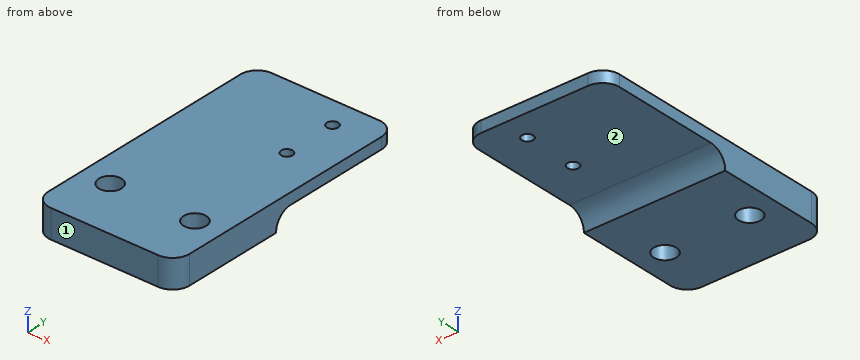
from build123d import *

# Parameters (mm, degrees)
SKETCH_1_W          = 25
SKETCH_1_H          = 46
EXTRUDE_1_DEPTH     = 5
SKETCH_2_W          = 25
SKETCH_2_H          = 25
CUT_EXTRUDE_1_DEPTH = 3
M4X0_7_1_D          = 4
M2X0_4_1_D          = 2
FILLET_1_R          = 3
FILLET_2_R          = 3


with BuildPart() as part:
    # ｽｹｯﾁ1 → ﾎﾞｽ - 押し出し1 (new body)
    with BuildSketch(Plane.XY):
        with Locations((12.5, 23)):
            Rectangle(SKETCH_1_W, SKETCH_1_H)
    extrude(amount=EXTRUDE_1_DEPTH)

    # ｽｹｯﾁ2 → ｶｯﾄ - 押し出し1 (cut)
    with BuildSketch(Plane(origin=(0, 0, 0), x_dir=(-1, 0, 0), z_dir=(0, 0, -1))):
        with Locations((-12.5, 33.5)):
            Rectangle(SKETCH_2_W, SKETCH_2_H)
    extrude(amount=-CUT_EXTRUDE_1_DEPTH, mode=Mode.SUBTRACT)

    # M4x0.7 ねじ穴1 (through all)
    with Locations(Plane.XY.offset(5)):
        with Locations((5, 10), (20, 10)):
            Hole(M4X0_7_1_D / 2)

    # M2x0.4 ねじ穴1 (through all)
    with Locations(Plane.XY.offset(5)):
        with Locations((18, 41), (18, 31.5)):
            Hole(M2X0_4_1_D / 2)

    # ﾌｨﾚｯﾄ1
    fillet_1_edges = [part.edges().sort_by_distance(p)[0] for p in [
        (12.5, 21, 3),
    ]]
    fillet(fillet_1_edges, radius=FILLET_1_R - 0.0001)  # a hair under: the kernel refuses the full size

    # ﾌｨﾚｯﾄ2
    fillet_2_edges = [part.edges().sort_by_distance(p)[0] for p in [
        (0, 46, 4),
        (25, 46, 4),
        (25, 0, 2.5),
        (0, 0, 2.5),
    ]]
    fillet(fillet_2_edges, radius=FILLET_2_R)


solid = part.part
Verification items for the finished model (mm, model axes). Face numbers are marked on the shaded views. A direction names the side the tool comes from. Coordinates: 2 decimals unless noted, no trailing zeros. Order: outer loops, then holes, each group sorted by start corner. A loop starts at its lowest first (then second) coordinate and runs counter-clockwise, first axis right, second up.
Item 1: Section check C-C, the plane y = 10. Enter the section's corners in (x, z).
Filled in:
outline: (0, 0) - (3, 0) - (3, 5) - (0, 5) - close; (7, 0) - (18, 0) - (18, 5) - (7, 5) - close; (22, 0) - (25, 0) - (25, 5) - (22, 5) - close
Item 2: Access from +Z, -Z, +X, -X, +Y, -Y to the whole of each face (thin tool, end or side, straight path). Record for the marked faces 1 and 2.
Filled in:
face 1: +Z, -Z, +X, -X, -Y
face 2: -Z, +X, -X, +Y
Item 3: Depth check by flat-ended pin: pin 1 (2.5 mm diameter, centred on x = 18, y = 31.5, fed in from -Z). Enter the tip coordinate at first touch or a pass-through.
Filled in:
pin 1: stops at z = 3
Item 4: Material ranges on L1, parallel to Y at x = 20.75, z = 4.3; L2, parallel to Z at x = 5, y = 31.5; L3, parallel to Y at x = 22.25, z = 2.5, recorded low to high.
Filled in:
L1: y = 0 to 8.15, 11.85 to 46
L2: z = 3 to 5
L3: y = 0.01 to 22.34
Item 5: Section check D-D, the plane z = 1.15. Enter the section's corners in (x, y), then the cut area to 3 significant figures.
Filled in:
outline: (0, 3) arc R3 ccw to (3, 0) - (22, 0) arc R3 ccw to (25, 3) - (25, 21.23) - (0, 21.23) - close; hole circle Ø4 at (5, 10); hole circle Ø4 at (20, 10)
area: 502 mm2
Item 6: Section check A-A, the plane y = 41. Enter the section's corners in (x, z).
Filled in:
outline: (0, 3) - (17, 3) - (17, 5) - (0, 5) - close; (19, 3) - (25, 3) - (25, 5) - (19, 5) - close
